Check sheet for the modelled part. Datum: model origin and axes. Units: mm. Give positions to 0.01 mm unless a question says otherwise; leave off trailing zeros. Order: outer loops, then holes, each group sorted by start corner. A loop starts at its lowest first (then second) coordinate and runs counter-clockwise, first axis right, second up. Notation, with made-up numbers: (-26, 40.5) -> (-8, 40.5) arc R30 ccw to (-8, 75.5) -> close; hole circle Ø8 at (65.5, -3.75). An arc over 180 degrees is marked (long way). Answer in a Markdown table with one row per item. Add a question column.
(1) Cross-section at B-B (y = 55). Record the cut outline in (x, z).
(2) Go/stop test with flat-tipped pins: pin 1 (1.5 mm diameter, centred on x = -21.5, z = -0.5, fed in from -Y); pin 2 (6 mm diameter, centred on x = -20, y = 70, fed in from -Z). Record where each tip stops, or that it passes through.
(3) Cross-section at C-C (z = -1.1). State how many separate pieces and enclosed holes the cut face has, then the cut area to 3 significant figures.
(4) Thickness scan on L1, parallel to Y at x = -20, z = -2.2; L2, parallel to Y at x = 5, z = -2.2; L3, parallel to Y at x = -24.5, z = -2.1. Record the ranges inside material, lowest first. Write a range as [from, to].
(5) Cross-section at A-A (x = -5). Record the cut outline in (y, z).
Autodesk Fusion 360 part; units mm, degrees
sketch "Sketch1" plane through (0, 0, 0) normal (0, 0, 1) x (1, 0, 0)
  line L0 (30, 80) -> (-30, 80)
  line L1 (-30, 80) -> (-30, -80)
  line L2 (-30, -80) -> (30, -80)
  line L3 (30, -80) -> (30, 80)
  line L4 (30, 80) -> (-30, -80) construction
  line L5 (-30, 80) -> (30, -80) construction
  line L6 (20, 70) -> (-20, 70) construction
  line L7 (-20, 70) -> (-20, -70) construction
  line L8 (-20, -70) -> (20, -70) construction
  line L9 (20, -70) -> (20, 70) construction
  line L10 (20, 70) -> (-20, -70) construction
  line L11 (-20, 70) -> (20, -70) construction
  line L12 (0, 0) -> (30, 0) construction
  circle A0 centre (20, 70) radius 2.25
  circle A1 centre (-20, 70) radius 2.25
  circle A2 centre (-20, -70) radius 2.25
  circle A3 centre (20, -70) radius 2.25
  line L13 (-30, 55) -> (30, 55) construction
  line L14 (0, 0) -> (0, 80) construction
  circle A4 centre (5, 55) radius 1.5
  circle A5 centre (-5, 55) radius 1.5
  circle A6 centre (5, -55) radius 1.5
  circle A7 centre (-5, -55) radius 1.5
  dimension "d1" = 160
  dimension "d2" = 60
  dimension "d3" = 40
  dimension "d4" = 140
  dimension "d5" = 4.5
  dimension "d6" = 4.5
  dimension "d11" = 3
  dimension "d12" = 5
  dimension "d13" = 55
extrude "Extrude1" add sketch "Sketch1" against normal blind 3
fillet "Fillet1" radius 10 4 edges at (-30, -80, -1.5) (30, -80, -1.5) (30, 80, -1.5) (-30, 80, -1.5)
equation "d6 = d5"
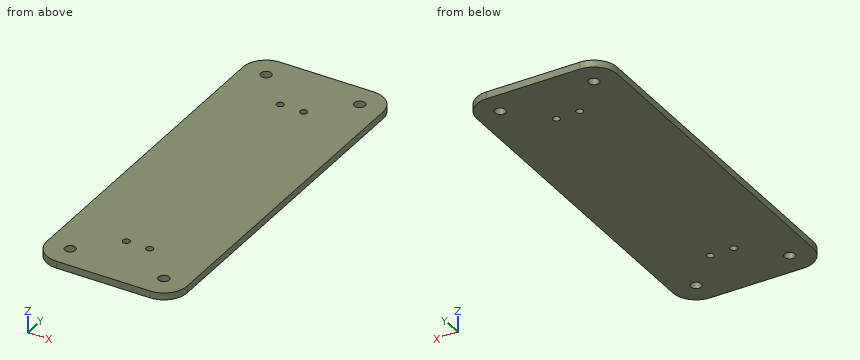
Answer below:
| question | item | result |
|---|---|---|
| 1 | outline | (-30, -3) -> (-6.5, -3) -> (-6.5, 0) -> (-30, 0) -> close; (-3.5, -3) -> (3.5, -3) -> (3.5, 0) -> (-3.5, 0) -> close; (6.5, -3) -> (30, -3) -> (30, 0) -> (6.5, 0) -> close |
| 2 | pin 1 | stops at y = -79.97 |
| 2 | pin 2 | stops at z = -3 |
| 3 | separate pieces | 1 |
| 3 | enclosed holes | 8 |
| 3 | area | 9,420 mm² |
| 4 | L1 | y = [-80, -72.25], [-67.75, 67.75], [72.25, 80] |
| 4 | L2 | y = [-80, -56.5], [-53.5, 53.5], [56.5, 80] |
| 4 | L3 | y = [-78.93, 78.93] |
| 5 | outline | (-80, -3) -> (-56.5, -3) -> (-56.5, 0) -> (-80, 0) -> close; (-53.5, -3) -> (53.5, -3) -> (53.5, 0) -> (-53.5, 0) -> close; (56.5, -3) -> (80, -3) -> (80, 0) -> (56.5, 0) -> close |
